from build123d import *

# Parameters (mm, degrees)
BOSS_EXTRUDE1_DEPTH             = 37
BOSS_EXTRUDE1_DEPTH_BACK        = 37
SKETCH2_W                       = 74
SKETCH2_H                       = 74
BOSS_EXTRUDE2_DEPTH             = 15
ADVANCEDHOLE1_START             = 20.194913472
ADVANCEDHOLE1_DEPTH             = 4.525323154
ADVANCEDHOLE1_START_2           = 14.194913472
ADVANCEDHOLE1_2_OUTLINE_R       = 3.2
ADVANCEDHOLE1_2_DEPTH           = 6
ADVANCEDHOLE2_START             = -24.720236626
ADVANCEDHOLE2_DEPTH             = 4.525323154
ADVANCEDHOLE2_START_2           = -20.194913472
ADVANCEDHOLE2_2_OUTLINE_R       = 3.2
ADVANCEDHOLE2_2_DEPTH           = 6
SKETCH11_W                      = 3
SKETCH11_H                      = 74
CUT_EXTRUDE1_DEPTH              = 1
M4_TAPPED_HOLE1_D               = 3.3
M4_TAPPED_HOLE1_DEPTH           = 10.1
M4_TAPPED_HOLE1_TIP             = 0.991420021
M4_TAPPED_HOLE1_ON_FACE_2_D     = 3.3
M4_TAPPED_HOLE1_ON_FACE_2_DEPTH = 10.1
M4_TAPPED_HOLE1_ON_FACE_2_TIP   = 0.991420021
M4_TAPPED_HOLE1_ON_FACE_3_D     = 3.3
M4_TAPPED_HOLE1_ON_FACE_3_DEPTH = 10.1
M4_TAPPED_HOLE1_ON_FACE_3_TIP   = 0.991420021
M4_TAPPED_HOLE1_ON_FACE_4_D     = 3.3
M4_TAPPED_HOLE1_ON_FACE_4_DEPTH = 10.1
M4_TAPPED_HOLE1_ON_FACE_4_TIP   = 0.991420021
CHAMFER1_SIZE                   = 4.2
CHAMFER2_SIZE                   = 1
CHAMFER2_SIZE2                  = 1.732050808
CUT_EXTRUDE2_DEPTH              = 74.199110283


# Read off the part's stored shape, not the designer's step: AdvancedHole1, AdvancedHole2
with BuildPart() as part:
    # Sketch1 → Boss-Extrude1 (new, two sides: drawn at the far end of the back side and taken through both)
    with BuildSketch(Plane(origin=(0, 0, 0), x_dir=(1, 0, 0), z_dir=(0, 1, 0)).offset(-BOSS_EXTRUDE1_DEPTH_BACK)):
        Polygon((-40, 2), (-48.436814511, 22.705321112), (-45.608387387, 25.533748237), (-23, 2.925360851), (-23, 2), (23, 2), (23, 2.925360851), (45.608387387, 25.533748237), (48.436814511, 22.705321112), (40, 2), (40, 0), (-40, 0), align=None)
    extrude(amount=BOSS_EXTRUDE1_DEPTH + BOSS_EXTRUDE1_DEPTH_BACK)

    # Sketch2 → Boss-Extrude2 (add)
    with BuildSketch(Plane.XY):
        Rectangle(SKETCH2_W, SKETCH2_H)
    extrude(amount=BOSS_EXTRUDE2_DEPTH)

    # AdvancedHole1 outline → AdvancedHole1 (cut)
    with BuildSketch(Plane(origin=(0, 0, 0), x_dir=(0.707106781186546, 0, -0.707106781186549), z_dir=(0.707106781186549, 0, 0.707106781186546)).offset(ADVANCEDHOLE1_START)):
        with BuildLine():
            Line((45.554363955, 28.35832814), (46.067784427, 30))
            Line((46.067784427, 30), (45.554363955, 31.64167186))
            ThreePointArc((45.554363955, 31.64167186), (34.805086528, 30), (45.554363955, 28.35832814))
        make_face()
        with BuildLine():
            ThreePointArc((45.554363955, -13.35832814), (34.805086528, -15), (45.554363955, -16.64167186))
            Line((45.554363955, -16.64167186), (46.067784427, -15))
            Line((46.067784427, -15), (45.554363955, -13.35832814))
        make_face()
    extrude(amount=ADVANCEDHOLE1_DEPTH, mode=Mode.SUBTRACT)

    # AdvancedHole1 2 outline → AdvancedHole1 2 (cut)
    with BuildSketch(Plane(origin=(0, 0, 0), x_dir=(0.707106781186546, 0, -0.707106781186549), z_dir=(0.707106781186549, 0, 0.707106781186546)).offset(ADVANCEDHOLE1_START_2)):
        with Locations((40.305086528, -15)):
            Circle(ADVANCEDHOLE1_2_OUTLINE_R)
        with Locations((40.305086528, 30)):
            Circle(ADVANCEDHOLE1_2_OUTLINE_R)
    extrude(amount=ADVANCEDHOLE1_2_DEPTH, mode=Mode.SUBTRACT)

    # AdvancedHole2 outline → AdvancedHole2 (cut)
    with BuildSketch(Plane(origin=(0, 0, 0), x_dir=(0.707106781186546, 0, 0.707106781186549), z_dir=(0.707106781186549, 0, -0.707106781186546)).offset(ADVANCEDHOLE2_START)):
        with BuildLine():
            Line((-46.067784427, 15), (-45.554363955, 13.35832814))
            ThreePointArc((-45.554363955, 13.35832814), (-34.805086528, 15), (-45.554363955, 16.64167186))
            Line((-45.554363955, 16.64167186), (-46.067784427, 15))
        make_face()
        with BuildLine():
            Line((-45.554363955, -28.35832814), (-46.067784427, -30))
            Line((-46.067784427, -30), (-45.554363955, -31.64167186))
            ThreePointArc((-45.554363955, -31.64167186), (-34.805086528, -30), (-45.554363955, -28.35832814))
        make_face()
    extrude(amount=ADVANCEDHOLE2_DEPTH, mode=Mode.SUBTRACT)

    # AdvancedHole2 2 outline → AdvancedHole2 2 (cut)
    with BuildSketch(Plane(origin=(0, 0, 0), x_dir=(0.707106781186546, 0, 0.707106781186549), z_dir=(0.707106781186549, 0, -0.707106781186546)).offset(ADVANCEDHOLE2_START_2)):
        with Locations((-40.305086528, 15)):
            Circle(ADVANCEDHOLE2_2_OUTLINE_R)
        with Locations((-40.305086528, -30)):
            Circle(ADVANCEDHOLE2_2_OUTLINE_R)
    extrude(amount=ADVANCEDHOLE2_2_DEPTH, mode=Mode.SUBTRACT)

    # Sketch11 → Cut-Extrude1 (cut)
    with BuildSketch(Plane.XY):
        with Locations((-38.5, 0)):
            Rectangle(SKETCH11_W, SKETCH11_H)
    extrude(amount=-CUT_EXTRUDE1_DEPTH, mode=Mode.SUBTRACT)

    # M4 Tapped Hole1
    with Locations(Plane(origin=(37, 29, 7.5), x_dir=(0, 0, 1), z_dir=(1, 0, 0))):
        with Locations((0, 0), (0, 58), (0, 29)):
            Hole(M4_TAPPED_HOLE1_D / 2, depth=M4_TAPPED_HOLE1_DEPTH)
            with Locations((0, 0, -(M4_TAPPED_HOLE1_DEPTH + M4_TAPPED_HOLE1_TIP / 2))):  # 118° drill point
                Cone(0, M4_TAPPED_HOLE1_D / 2, M4_TAPPED_HOLE1_TIP, mode=Mode.SUBTRACT)

    # M4 Tapped Hole1 on face 2
    with Locations(Plane(origin=(-37, 29, 7.5), x_dir=(0, 0, -1), z_dir=(-1, 0, 0))):
        with Locations((0, 0), (0, 58), (0, 29)):
            Hole(M4_TAPPED_HOLE1_ON_FACE_2_D / 2, depth=M4_TAPPED_HOLE1_ON_FACE_2_DEPTH)
            with Locations((0, 0, -(M4_TAPPED_HOLE1_ON_FACE_2_DEPTH + M4_TAPPED_HOLE1_ON_FACE_2_TIP / 2))):  # 118° drill point
                Cone(0, M4_TAPPED_HOLE1_ON_FACE_2_D / 2, M4_TAPPED_HOLE1_ON_FACE_2_TIP, mode=Mode.SUBTRACT)

    # M4 Tapped Hole1 on face 3
    with Locations(Plane(origin=(21, 37, 7.5), x_dir=(0, 0, 1), z_dir=(0, 1, 0))):
        with Locations((0, 0), (0, -42)):
            Hole(M4_TAPPED_HOLE1_ON_FACE_3_D / 2, depth=M4_TAPPED_HOLE1_ON_FACE_3_DEPTH)
            with Locations((0, 0, -(M4_TAPPED_HOLE1_ON_FACE_3_DEPTH + M4_TAPPED_HOLE1_ON_FACE_3_TIP / 2))):  # 118° drill point
                Cone(0, M4_TAPPED_HOLE1_ON_FACE_3_D / 2, M4_TAPPED_HOLE1_ON_FACE_3_TIP, mode=Mode.SUBTRACT)

    # M4 Tapped Hole1 on face 4
    with Locations(Plane(origin=(-21, -37, 7.5), x_dir=(0, 0, -1), z_dir=(0, -1, 0))):
        with Locations((0, 0), (0, 42)):
            Hole(M4_TAPPED_HOLE1_ON_FACE_4_D / 2, depth=M4_TAPPED_HOLE1_ON_FACE_4_DEPTH)
            with Locations((0, 0, -(M4_TAPPED_HOLE1_ON_FACE_4_DEPTH + M4_TAPPED_HOLE1_ON_FACE_4_TIP / 2))):  # 118° drill point
                Cone(0, M4_TAPPED_HOLE1_ON_FACE_4_D / 2, M4_TAPPED_HOLE1_ON_FACE_4_TIP, mode=Mode.SUBTRACT)

    # Chamfer1
    chamfer1_edges = [part.edges().sort_by_distance(p)[0] for p in [
        (37, -37, 7.5),
        (37, 37, 7.5),
        (-37, 37, 7),
        (-37, -37, 7),
    ]]
    chamfer(chamfer1_edges, length=CHAMFER1_SIZE)

    # Chamfer2
    chamfer2_edges = [part.edges().sort_by_distance(p)[0] for p in [
        (37, 0, 15),
        (0, -37, 15),
        (0, 37, 15),
        (-37, 0, 15),
        (34.9, 34.9, 15),
        (-34.9, 34.9, 15),
        (-34.9, -34.9, 15),
        (34.9, -34.9, 15),
    ]]
    chamfer2_side = [part.faces().sort_by_distance(p)[0] for p in [
        (0, 0, 15),
    ]]
    chamfer(chamfer2_edges, length=CHAMFER2_SIZE, length2=CHAMFER2_SIZE2, reference=chamfer2_side[0])

    # Sketch13 → Cut-Extrude2 (cut, through all)
    with BuildSketch(Plane.XY.offset(15)):
        with BuildLine():
            Line((-21, 17), (-21, -17))
            ThreePointArc((-21, -17), (-19.828427125, -19.828427125), (-17, -21))
            Line((-17, -21), (17, -21))
            ThreePointArc((17, -21), (19.828427125, -19.828427125), (21, -17))
            Line((21, -17), (21, 17))
            ThreePointArc((21, 17), (19.828427125, 19.828427125), (17, 21))
            Line((17, 21), (-17, 21))
            ThreePointArc((-17, 21), (-19.828427125, 19.828427125), (-21, 17))
        make_face()
    extrude(amount=-CUT_EXTRUDE2_DEPTH, mode=Mode.SUBTRACT)


solid = part.part
Input: part model. Units: mm. Frame: model coordinates. A direction names the side the tool comes from. Coordinates: 2 decimals unless noted, no trailing zeros. Order: outer loops, then holes, each group sorted by start corner. A loop starts at its lowest first (then second) coordinate and runs counter-clockwise, first axis right, second up. Notation, with made-up numbers: M 64,51.5 L 123,51.5 A29 ccw 123,85.5 Z; hole C 85.5,-23.75 d8. An arc over 180 degrees is marked long. Write item = value, one per line. Start each with the question number.
(1) Section C-C on z = 3. Output: boundary loops of the cut face in (x, y), and give its area (3 significant figures).
(2) Section D-D on z = -6. Output: boundary loops of the cut face in (x, y), and give its area (3 significant figures).
(3) Pull-direction query (Y, two-part tool) for faces 1 (the flat face through (34.522, 34.581, 14.122)), 2 (the flat face through (37, 0, 5)), 3 (the cylindrical face through (40.12, 30.22, -9.11)); classes: released by +Y, released by -Y, zero draft, split by the parting line, or undercut.
(4) First-contact query: P1, Ø18.5, axis at y = -8, z = 9, coming from the -X side; P2, Ø14, axis at x = -10, y = -3, coming from the -Z side; P3, Ø6, axis at y = 21.5, z = 9, coming from the +X side; P4, Ø3, axis at y = 12.5, z = -16.5, coming from the +X side. Flat tips, straight axial feed; report the tip coordinate or a pass-through.
(5) Section B-B on y = 9. Output: boundary loops of the cut face in (x, z), and give its area (3 significant figures).
(6) Line query: line 1 along X through (y, z) = (-33.5, 7.5); line 2 along Y through (x, z) = (32.75, 7.5); line 3 along Z through (x, y) = (21, -31). Output: solid intervals per line, ascending. Write a range as [from, to].
(7) Reachability of faces 4 (the cylindrical face through (22.636, 31.879, 7.715)), 5 (the flat face through (34.9, 34.9, 6.5)), 6 (the flat face through (-34.462, -0.518, -14.388)), 7 (the cylindrical face through (19.859, 19.797, 6.619)), 8 (the cylindrical face through (-31.879, -30.636, 7.285)) from +Z, -Z, +X, -X, +Y, -Y: full face, straight path, thin tool, end or side. Return the list, or none.
(8) Section A-A on x = -7. Output: boundary loops of the cut face in (y, z), and give its area (3 significant figures).
Result set:
q1.outline = M -37,-32.8 L -32.8,-37 L 32.8,-37 L 37,-32.8 L 37,32.8 L 32.8,37 L -32.8,37 L -37,32.8 Z; hole M -21,-17 A4 ccw -17,-21 L 17,-21 A4 ccw 21,-17 L 21,17 A4 ccw 17,21 L -17,21 A4 ccw -21,17 Z
q1.area = 3,690 mm²
q2.outline = M -41.63,-37 L -26.07,-37 L -26.07,37 L -41.63,37 Z; M 26.07,-37 L 41.63,-37 L 41.63,37 L 26.07,37 Z
q2.area = 2,300 mm²
q3.face_1 = released by +Y
q3.face_2 = zero draft
q3.face_3 = undercut
q4.P1 = -37
q4.P2 = through
q4.P3 = 37
q4.P4 = 46.52
q5.outline = M -48.44,-22.71 L -45.61,-25.53 L -23,-2.93 L -23,-2 L -21,-2 L -21,15 L -36,15 L -37,13.27 L -37,-1 L -40,-1 L -40,-2 Z; M 21,-2 L 23,-2 L 23,-2.93 L 45.61,-25.53 L 48.44,-22.71 L 40,-2 L 40,0 L 37,0 L 37,13.27 L 36,15 L 21,15 Z
q5.area = 1,050 mm²
q6.line_1 = [-36.3, -22.65], [-19.35, 19.35], [22.65, 36.3]
q6.line_2 = [-37, -30.65], [-27.35, -1.65], [1.65, 27.35], [30.65, 37]
q6.line_3 = [-2, 5.85], [9.15, 15]
q7.face_4 = +Y
q7.face_5 = +Z, +X, +Y
q7.face_6 = -Z, +Y, -Y
q7.face_7 = +Z, -Z
q7.face_8 = -X
q8.outline = M -37,-2 L -21,-2 L -21,15 L -36,15 L -37,13.27 Z; M 21,-2 L 37,-2 L 37,13.27 L 36,15 L 21,15 Z
q8.area = 542 mm²
